Here's how the part is built. I have some questions about the finished solid (model axes, mm). A direction names the side the tool comes from. Round coordinates to 2 decimals unless told otherwise and drop trailing zeros. Order: outer loops, then holes, each group sorted by start corner. A loop starts at its lowest first (then second) coordinate and runs counter-clockwise, first axis right, second up. Notation, with made-up numbers: (89, 13.5) -> (142, 13.5) arc R14 ccw to (142, 36.5) -> close; hole circle Ø1 at (72, 9.25). An arc over 180 degrees is marked (long way). Use a Markdown table: item, result. Add a question column.
(1) If I drill on probe 1 along Y at (x, z) = (0, 302); probe 2 along Z at (x, y) = (1.75, 1.5); probe 3 along Z at (x, y) = (3.75, -4.5), over which ranges is the centre line in solid material (lowest first)?
(2) I'm going to push flat-ended pins straight in: P1, Ø5, axis at y = 8, z = 264, coming from the -X side; P2, Ø6, axis at y = -8, z = 128, coming from the +X side; P3, Ø4, axis at x = 5.5, z = 287, coming from the -Y side. Where does each tip first touch, or does it pass through?
(3) I want a section at C-C, the plane z = 57. Please give me the cut outline in (x, y).
(4) On a 3-axis mill with a long thin cutter (end or side, diameter ignored), from which of +Z, -Z, +X, -X, +Y, -Y can I reach the whole of each face in a straight line? I mean faces 1 (the face through (0, 0, 0)), 2 (the face through (-1.08, -4.88, 314.72)). Say none if no direction works.
(5) I want a section at A-A, the plane x = 0. Please give me the cut outline in (y, z), then the cut area to 3 significant figures.
(6) Thinking about a two-plate mould opening in X: for faces 3 (the face through (0, 0, 290)), 4 (the face through (6.2, -2, 340)), 5 (the face through (-1.4, 10.66, 167)), which applies, pulls with the +X half, pulls with the -X half, needs draft (parallel to the pull), parting line crosses it, or undercut?
from build123d import *

# Parameters (mm, degrees)
SKETCH1_R           = 2.15
BOSS_EXTRUDE1_DEPTH = 68
SKETCH2_R           = 1
CUT_EXTRUDE1_DEPTH  = 10
FILLET1_R           = 0.25
SCALE1_SCALE        = 5


with BuildPart() as part:
    # Sketch1 → Boss-Extrude1 (new body)
    with BuildSketch(Plane.XY):
        Circle(SKETCH1_R)
    extrude(amount=BOSS_EXTRUDE1_DEPTH)

    # Sketch2 → Cut-Extrude1 (cut)
    with BuildSketch(Plane.XY.offset(68)):
        Circle(SKETCH2_R)
    extrude(amount=-CUT_EXTRUDE1_DEPTH, mode=Mode.SUBTRACT)

    # Fillet1
    fillet1_edges = [part.edges().sort_by_distance(p)[0] for p in [
        (-2.15, 0, 68),
        (-1, 0, 68),
    ]]
    fillet(fillet1_edges, radius=FILLET1_R)


with BuildPart() as part_1:
    # Scale1: scaled about (0, 0, 0)
    add(part.part.scale(SCALE1_SCALE))


solid = part_1.part
Taken from the geometry:
| question | item | result |
|---|---|---|
| 1 | probe 1 | y = -10.75 to -5, 5 to 10.75 |
| 1 | probe 2 | z = 0 to 290 |
| 1 | probe 3 | z = 0 to 339.94 |
| 2 | P1 | stops at x = -9.24 |
| 2 | P2 | stops at x = 9.52 |
| 2 | P3 | stops at y = -10.16 |
| 3 | outline | circle Ø21.5 at (0, 0) |
| 4 | face 1 | -Z, +X, -X, +Y, -Y |
| 4 | face 2 | +Z |
| 5 | outline | (-10.75, 0) -> (10.75, 0) -> (10.75, 338.75) arc R1.25 ccw to (9.5, 340) -> (6.25, 340) arc R1.25 ccw to (5, 338.75) -> (5, 290) -> (-5, 290) -> (-5, 338.75) arc R1.25 ccw to (-6.25, 340) -> (-9.5, 340) arc R1.25 ccw to (-10.75, 338.75) -> close |
| 5 | area | 6,810 mm2 |
| 6 | face 3 | undercut |
| 6 | face 4 | needs draft |
| 6 | face 5 | parting line crosses it |
